```python
from build123d import *

# Parameters (mm, degrees)
BOSS_EXTRUDE1_DEPTH      = 22
BOSS_EXTRUDE1_DEPTH_BACK = 22
SKETCH2_W                = 38
SKETCH2_H                = 20
CUT_EXTRUDE1_DEPTH       = 105.423416914
SKETCH3_W                = 7
SKETCH3_H                = 44
BOSS_EXTRUDE2_DEPTH      = 65.5
SKETCH23_R               = 5
SKETCH23_R_2             = 1.2
CUT_EXTRUDE2_DEPTH       = 111.605436123
SKETCH24_W               = 28.5
SKETCH24_H               = 34
CUT_EXTRUDE3_DEPTH       = 90.954502389
SKETCH26_R               = 1.2
SKETCH26_R_2             = 5
SKETCH26_R_3             = 1.45
CUT_EXTRUDE6_DEPTH       = 107.330263801
SKETCH27_W               = 29.7
SKETCH27_H               = 35.2
CUT_EXTRUDE8_DEPTH       = 73.137455597
SKETCH29_W               = 7
SKETCH29_H               = 35
CUT_EXTRUDE10_DEPTH      = 74.468530678
CHAMFER2_SIZE            = 5
FILLET1_START            = -23
FILLET1_DEPTH            = 46
FILLET2_R                = 10


with BuildPart() as part:
    # Sketch1 → Boss-Extrude1 (new, two sides: drawn at the far end of the back side and taken through both)
    with BuildSketch(Plane.XY.offset(-BOSS_EXTRUDE1_DEPTH_BACK)):
        with BuildLine():
            Line((10.25, -60), (10.25, 0))
            ThreePointArc((10.25, 0), (0, -10.25), (-10.25, 0))
            Line((-10.25, 0), (-10.25, -60))
            Line((-10.25, -60), (-10.25, -100))
            Line((-10.25, -100), (10.25, -100))
            Line((10.25, -100), (10.25, -60))
        make_face()
        with BuildLine():
            Line((10.25, 0), (9.2, 0))
            ThreePointArc((9.2, 0), (8.816088231, -0.879772698), (7.91, -1.196620241))
            ThreePointArc((7.91, -1.196620241), (5.656854249, -5.656854249), (1.196620241, -7.91))
            ThreePointArc((1.196620241, -7.91), (1.199154762, -7.954968281), (1.2, -8))
            ThreePointArc((1.2, -8), (-0.045031719, -9.199154762), (-1.196620241, -7.91))
            ThreePointArc((-1.196620241, -7.91), (-5.656854249, -5.656854249), (-7.91, -1.196620241))
            ThreePointArc((-7.91, -1.196620241), (-8.816088231, -0.879772698), (-9.2, 0))
            Line((-9.2, 0), (-10.25, 0))
            ThreePointArc((-10.25, 0), (0, -10.25), (10.25, 0))
        make_face()
        with BuildLine():
            ThreePointArc((7.91, -1.196620241), (7.120227302, -0.816088231), (6.8, 0))
            Line((6.8, 0), (4.2, 0))
            ThreePointArc((4.2, 0), (0, -4.2), (-4.2, 0))
            Line((-4.2, 0), (-6.8, 0))
            ThreePointArc((-6.8, 0), (-7.120227302, -0.816088231), (-7.91, -1.196620241))
            ThreePointArc((-7.91, -1.196620241), (-5.656854249, -5.656854249), (-1.196620241, -7.91))
            ThreePointArc((-1.196620241, -7.91), (0, -6.8), (1.196620241, -7.91))
            ThreePointArc((1.196620241, -7.91), (5.656854249, -5.656854249), (7.91, -1.196620241))
        make_face()
        with BuildLine():
            Line((4.2, 0), (6.8, 0))
            ThreePointArc((6.8, 0), (7.120227302, 0.816088231), (7.91, 1.196620241))
            ThreePointArc((7.91, 1.196620241), (5.656854249, 5.656854249), (1.196620241, 7.91))
            ThreePointArc((1.196620241, 7.91), (0, 6.8), (-1.196620241, 7.91))
            ThreePointArc((-1.196620241, 7.91), (-5.656854249, 5.656854249), (-7.91, 1.196620241))
            ThreePointArc((-7.91, 1.196620241), (-7.120227302, 0.816088231), (-6.8, 0))
            Line((-6.8, 0), (-4.2, 0))
            ThreePointArc((-4.2, 0), (0, 4.2), (4.2, 0))
        make_face()
        with BuildLine():
            ThreePointArc((7.91, 1.196620241), (8.816088231, 0.879772698), (9.2, 0))
            Line((9.2, 0), (10.25, 0))
            ThreePointArc((10.25, 0), (0, 10.25), (-10.25, 0))
            Line((-10.25, 0), (-9.2, 0))
            ThreePointArc((-9.2, 0), (-8.816088231, 0.879772698), (-7.91, 1.196620241))
            ThreePointArc((-7.91, 1.196620241), (-5.656854249, 5.656854249), (-1.196620241, 7.91))
            ThreePointArc((-1.196620241, 7.91), (-0.045031719, 9.199154762), (1.2, 8))
            ThreePointArc((1.2, 8), (1.199154762, 7.954968281), (1.196620241, 7.91))
            ThreePointArc((1.196620241, 7.91), (5.656854249, 5.656854249), (7.91, 1.196620241))
        make_face()
    extrude(amount=BOSS_EXTRUDE1_DEPTH + BOSS_EXTRUDE1_DEPTH_BACK)

    # Sketch2 → Cut-Extrude1 (cut, through all)
    with BuildSketch(Plane.ZY.offset(10.25)):
        with Locations((0, 0.25)):
            Rectangle(SKETCH2_W, SKETCH2_H)
    extrude(amount=-CUT_EXTRUDE1_DEPTH, mode=Mode.SUBTRACT)

    # Sketch3 → Boss-Extrude2 (add)
    with BuildSketch(Plane(origin=(0, -9.75, 0), x_dir=(1, 0, 0), z_dir=(0, 1, 0))):
        with Locations((-13.75, 0)):
            Rectangle(SKETCH3_W, SKETCH3_H)
        with Locations((13.75, 0)):
            Rectangle(SKETCH3_W, SKETCH3_H)
    extrude(amount=-BOSS_EXTRUDE2_DEPTH)

    # Sketch23 → Cut-Extrude2 (cut, through all)
    with BuildSketch(Plane.XY.offset(22)):
        with BuildLine():
            Line((-10.25, -100), (10.25, -100))
            Line((10.25, -100), (10.25, -85))
            ThreePointArc((10.25, -85), (0, -95.25), (-10.25, -85))
            Line((-10.25, -85), (-10.25, -100))
        make_face()
        with Locations((0, -85)):
            Circle(SKETCH23_R)
        with Locations((8, -85)):
            Circle(SKETCH23_R_2)
        with Locations((0, -77)):
            Circle(SKETCH23_R_2)
        with Locations((0, -93)):
            Circle(SKETCH23_R_2)
        with Locations((-8, -85)):
            Circle(SKETCH23_R_2)
    extrude(amount=-CUT_EXTRUDE2_DEPTH, mode=Mode.SUBTRACT)

    # Sketch24 → Cut-Extrude3 (cut, through all)
    with BuildSketch(Plane(origin=(0, -9.75, 0), x_dir=(1, 0, 0), z_dir=(0, 1, 0))):
        Rectangle(SKETCH24_W, SKETCH24_H)
    extrude(amount=-CUT_EXTRUDE3_DEPTH, mode=Mode.SUBTRACT)

    # Sketch26 → Cut-Extrude6 (cut, through all)
    # profile 1 of 5: a face of its own
    with BuildSketch(Plane.XY.offset(22)):
        with BuildLine():
            Line((10.25, -75.25), (14.25, -75.25))
            Line((14.25, -75.25), (14.25, -56.53282359))
            Line((14.25, -56.53282359), (14.25, -56.25))
            Line((14.25, -56.25), (-14.25, -56.25))
            Line((-14.25, -56.25), (-14.25, -56.53282359))
            Line((-14.25, -56.53282359), (-14.25, -75.25))
            Line((-14.25, -75.25), (-10.25, -75.25))
            Line((-10.25, -75.25), (-10.25, -85))
            ThreePointArc((-10.25, -85), (0, -95.25), (10.25, -85))
            Line((10.25, -85), (10.25, -75.25))
        make_face()
        with Locations((-8, -85)):
            Circle(SKETCH26_R, mode=Mode.SUBTRACT)
        with Locations((0, -85)):
            Circle(SKETCH26_R_2, mode=Mode.SUBTRACT)
        with Locations((0, -77)):
            Circle(SKETCH26_R, mode=Mode.SUBTRACT)
        with Locations((0, -93)):
            Circle(SKETCH26_R, mode=Mode.SUBTRACT)
        with Locations((8, -85)):
            Circle(SKETCH26_R, mode=Mode.SUBTRACT)
    # profile 2 of 5: a face of its own
    with BuildSketch(Plane.XY.offset(22)):
        Polygon((-17.25, -75.25), (-14.25, -75.25), (-14.25, -56.53282359), (-14.25, -56.25), (-17.25, -56.25), align=None)
    # profile 3 of 5: a face of its own
    with BuildSketch(Plane.XY.offset(22)):
        Polygon((14.25, -56.53282359), (14.25, -75.25), (17.25, -75.25), (17.25, -56.25), (14.25, -56.25), align=None)
    # profile 4 of 5: a face of its own
    with BuildSketch(Plane.XY.offset(22)):
        with Locations((-11, -53)):
            Circle(SKETCH26_R_3)
    # profile 5 of 5: a face of its own
    with BuildSketch(Plane.XY.offset(22)):
        with Locations((11, -53)):
            Circle(SKETCH26_R_3)
    extrude(amount=-CUT_EXTRUDE6_DEPTH, mode=Mode.SUBTRACT)

    # Sketch27 → Cut-Extrude8 (cut, through all)
    with BuildSketch(Plane.XZ.offset(56.25)):
        Rectangle(SKETCH27_W, SKETCH27_H)
    extrude(amount=-CUT_EXTRUDE8_DEPTH, mode=Mode.SUBTRACT)

    # Sketch29 → Cut-Extrude10 (cut, through all)
    with BuildSketch(Plane(origin=(0, 0, -22), x_dir=(-1, 0, 0), z_dir=(0, 0, -1))):
        with Locations((-13.75, -27.25)):
            Rectangle(SKETCH29_W, SKETCH29_H)
    extrude(amount=-CUT_EXTRUDE10_DEPTH, mode=Mode.SUBTRACT)

    # Chamfer2
    # the kernel refuses this chamfer: 5 mm, written as the material it takes off along each edge
    with BuildSketch(Plane(origin=(-17.25, -56.25, 34.85841494), x_dir=(1, 0, 0), z_dir=(0, 0, -1))) as chamfer2_piece_1:
        Polygon((CHAMFER2_SIZE, 0), (0, -CHAMFER2_SIZE), (0, 0), align=None)
    extrude(amount=69.71682988, mode=Mode.SUBTRACT)

    # Fillet1: read off the stored shape, not the designer's step
    # Fillet1 outline → Fillet1 (cut)
    with BuildSketch(Plane.XY.offset(FILLET1_START)):
        with BuildLine():
            ThreePointArc((10.25, -44.75), (15.312257748, -48.373312231), (17.25, -54.289392014))
            Line((17.25, -54.289392014), (17.25, -44.75))
            Line((17.25, -44.75), (10.25, -44.75))
        make_face()
    extrude(amount=FILLET1_DEPTH, mode=Mode.SUBTRACT)

    # Fillet2
    # the kernel refuses this fillet: 10 mm, written as the material it takes off along each edge
    with BuildSketch(Plane(origin=(-17.25, -9.75, -47), x_dir=(1, 0, 0), z_dir=(0, 0, 1))) as fillet2_piece_1_section:
        with BuildLine():
            CenterArc((FILLET2_R, -FILLET2_R), FILLET2_R, 90, 90)
            Line((0, -FILLET2_R), (0, 0))
            Line((0, 0), (FILLET2_R, 0))
        make_face()
    fillet2_piece_1 = extrude(amount=94, mode=Mode.PRIVATE)
    fillet2_piece_1 = split(fillet2_piece_1, bisect_by=Plane(origin=(-10.25, -9.75, -47), z_dir=(-1, 0, 0)), keep=Keep.TOP, mode=Mode.PRIVATE)
    add(fillet2_piece_1, mode=Mode.SUBTRACT)
    with BuildSketch(Plane(origin=(-17.25, -9.75, -47), x_dir=(1, 0, 0), z_dir=(0, 0, 1))) as fillet2_piece_2_section:
        with BuildLine():
            CenterArc((FILLET2_R, -FILLET2_R), FILLET2_R, 90, 90)
            Line((0, -FILLET2_R), (0, 0))
            Line((0, 0), (FILLET2_R, 0))
        make_face()
    fillet2_piece_2 = extrude(amount=94, mode=Mode.PRIVATE)
    fillet2_piece_2 = split(fillet2_piece_2, bisect_by=Plane(origin=(-17.25, -9.75, -19), z_dir=(0, 0, 1)), keep=Keep.TOP, mode=Mode.PRIVATE)
    fillet2_piece_2 = split(fillet2_piece_2, bisect_by=Plane(origin=(-17.25, -9.75, 19), z_dir=(0, 0, -1)), keep=Keep.TOP, mode=Mode.PRIVATE)
    add(fillet2_piece_2, mode=Mode.SUBTRACT)


solid = part.part
```
Here's how the part is built. I have some questions about the finished solid (model axes, mm). A direction names the side the tool comes from. Give positions to 0.01 mm unless a question says otherwise; leave off trailing zeros. Write each loop counter-clockwise with the first axis right and the second up, starting at its lowest first coordinate (ties: lowest second). Pieces come first, ordered by that corner, then holes.
(1) Imagine slicing it at D-D, the plane y = -22.5. Write out the boundary of the cut face in (x, z), and give its area (3 significant figures).
Output values:
outline: (-17.25, -22) - (10.25, -22) - (10.25, -17.6) - (-14.85, -17.6) - (-14.85, 17.6) - (10.25, 17.6) - (10.25, 22) - (-17.25, 22) - close
area: 326 mm2
(2) On a 3-axis mill with a long thin cutter (end or side, diameter ignored), from which of +Z, -Z, +X, -X, +Y, -Y can I reach the whole of each face in a straight line? I mean faces 4 (the face through (0, -33, -17.6)), 5 (the face through (10.25, -23, 20)), 6 (the face through (-10.25, -5, -20)). Say none if no direction works.
Output values:
face 4: +Y, -Y
face 5: +Z, -Z, +X, +Y
face 6: +Z, -Z, -X, +Y
(3) Thinking about a two-plate mould opening in Y: for faces 1 (the face through (10.686, -54.416, 19.831)), 2 (the face through (-4, -30, -22)), 3 (the face through (0.225, 10.248, 20.479)), which applies, pulls with the +Y half, pulls with the -Y half, needs draft (parallel to the pull), parting line crosses it, or undercut?
Output values:
face 1: undercut
face 2: needs draft
face 3: pulls with the +Y half
(4) If I drill on L1, parallel to Z at x = 3, y = -49.5; L2, parallel to Z at x = 7, y = 6; L3, parallel to X at y = -39.5, z = 1, over which ranges is the centre line in solid material (lowest first)?
Output values:
L1: z = -22 to -17.6, 17.6 to 22
L2: z = -22 to -19, 19 to 22
L3: x = -17.25 to -14.85
(5) Imagine slicing it at B-B, the plane y = -5. Write out the boundary of the cut face in (x, z), and give its area (3 significant figures).
Output values:
outline: (-10.25, -22) - (10.25, -22) - (10.25, -19) - (-10.25, -19) - close; (-10.25, 19) - (10.25, 19) - (10.25, 22) - (-10.25, 22) - close
area: 123 mm2
(6) Imagine slicing it at A-A, the plane z = 1. Write out the boundary of the cut face in (x, y).
Output values:
outline: (-17.25, -51.25) - (-14.85, -53.65) - (-14.85, -13.25) arc R10 ccw to (-17.25, -19.75) - close; (14.85, -56.25) - (17.25, -56.25) - (17.25, -54.29) arc R10 ccw to (14.85, -47.79) - close
(7) Imagine slicing it at C-C, the plane x = 11. Write out the boundary of the cut face in (y, z), and give its area (3 significant figures).
Output values:
outline: (-56.25, -22) - (-54.45, -22) - (-54.45, -17.6) - (-56.25, -17.6) - close; (-56.25, 17.6) - (-54.45, 17.6) - (-54.45, 22) - (-56.25, 22) - close; (-51.55, -22) - (-45.02, -22) - (-45.02, -17.6) - (-51.55, -17.6) - close; (-51.55, 17.6) - (-45.02, 17.6) - (-45.02, 22) - (-51.55, 22) - close
area: 73.3 mm2
(8) Will these pins go through, and if not, where does the flat tip stop? pin 1 (3.5 mm diameter, centred on y = -6, z = -20.5, fed in from -X); pin 2 (3 mm diameter, centred on y = -47, z = 6.5, fed in from +X); pin 3 (4 mm diameter, centred on x = 12.5, z = 16.5, fed in from -Y); pin 4 (2.5 mm diameter, centred on x = 11, y = -53, fed in from +Z).
Output values:
pin 1: stops at x = -10.25
pin 2: stops at x = 15.4
pin 3: stops at y = -56.25
pin 4: passes through
